Work out the finished part from the listing and answer in its coordinate system (mm). A direction names the side the tool comes from. Give positions to 0.01 mm unless a question says otherwise; leave off trailing zeros. Write each loop counter-clockwise with the first axis right and the second up, starting at its lowest first coordinate (ties: lowest second). Pieces come first, ordered by that corner, then holes. Notation, with made-up numbers: (19, -17) -> (39, -17) arc R27 cw to (39, 8) -> close; hole circle Ø2 at (59, 82). An arc over 180 degrees is marked (long way). Use a Markdown table: item, result. Add a question column.
Q1. For faces 1 (the face through (10.1, 1, 5)), 2 (the face through (12, -1, 10)), 3 (the face through (13.1, -1, 5)), 4 (the face through (-26.58, 5.75, 12.07)), 5 (the face through (-37, 38, 5)), determine the directions among +Z, -Z, +X, -X, +Y, -Y from which every point of the face is accessible in a straight line to the end or side of a thin tool.
Q2. Each of these flat-tipped pins is pushed along its axis until it touches: pin 1 Ø7 at (y, z) = (4, 14) entering from +X; pin 2 Ø4 at (y, z) = (5.1, 15) entering from -X; pin 3 Ø2 at (y, z) = (1, 4.5) entering from -X; pin 4 Ø12 at (y, z) = (40.5, 14.5) entering from -X. Where does it stop, or does it pass through?
Q3. For a pull along Z with two mould halves and no side action, classify faces 6 (the face through (-31.88, 4.56, 18.26)), 7 (the face through (-9.37, 5.17, 16.6)), 8 (the face through (-19, 3.8, 13.7)), 9 (the face through (5, 0, 8)) as pulls with the +Z half, pulls with the -Z half, needs draft (parallel to the pull), parting line crosses it, or undercut.
Q4. Section B-B, the plane x = -27 is taken. Give the vertices of the cut face in (y, z), plus the area to 3 significant figures.
Q5. Consider line 1 (Z direction, x = -23.5, y = 5.1); line 2 (Z direction, x = -6, y = 5); line 3 (Y direction, x = -9.75, z = 15). Determine where each line is inside the solid, lowest interval first.
Q6. Section A-A, the plane z = 6.25 is taken. Give the vertices of the cut face in (x, y), plus the area to 3 significant figures.
Q7. Section D-D, the plane z = 15 is taken. Give the vertices of the cut face in (x, y).
from build123d import *

# Parameters (mm, degrees)
EXTRUDE_1_DEPTH     = 10
SKETCH_2_W          = 30.142135624
SKETCH_2_H          = 14
EXTRUDE_2_DEPTH     = 10
CHAMFER_2_SIZE      = 10
SKETCH_3_R          = 1.6
CUT_EXTRUDE_1_DEPTH = 77.000065789
SKETCH_4_R          = 3
CUT_EXTRUDE_2_DEPTH = 23


with BuildPart() as part:
    # ｽｹｯﾁ1 → ﾎﾞｽ - 押し出し1 (new body)
    with BuildSketch(Plane.XY):
        Polygon((0, 0), (0, 10.1), (-30, 10.1), (-37, 17.1), (-37, 60.1), (-42, 60.1), (-42, 7.957864376), (-30.142135624, -3.9), (13.1, -3.9), (13.1, 2), (10.1, 2), (10.1, 0), align=None)
    extrude(amount=EXTRUDE_1_DEPTH)

    # ｽｹｯﾁ2 → ﾎﾞｽ - 押し出し2 (add)
    with BuildSketch(Plane.XY.offset(10)):
        with Locations((-15.071067812, 3.1)):
            Rectangle(SKETCH_2_W, SKETCH_2_H)
    extrude(amount=EXTRUDE_2_DEPTH)

    # 面取り2
    chamfer_2_edges = [part.edges().sort_by_distance(p)[0] for p in [
        (-30.142135624, 3.1, 10),
        (0, -1.95, 10),
    ]]
    chamfer(chamfer_2_edges, length=CHAMFER_2_SIZE - 0.0001)  # a hair under: the kernel refuses the full size

    # ｽｹｯﾁ3 → ｶｯﾄ - 押し出し1 (cut, through all)
    with BuildSketch(Plane(origin=(0, 0, 0), x_dir=(0, 0, -1), z_dir=(1, 0, 0))):
        with Locations((-15, 5.1)):
            Circle(SKETCH_3_R)
    extrude(amount=-CUT_EXTRUDE_1_DEPTH, mode=Mode.SUBTRACT)

    # ｽｹｯﾁ4 → ｶｯﾄ - 押し出し2 (cut)
    with BuildSketch(Plane.ZY.offset(42)):
        with Locations(Location((15, 5.1, 0), (0, 0, 270))):
            Circle(SKETCH_4_R)
    extrude(amount=-CUT_EXTRUDE_2_DEPTH, mode=Mode.SUBTRACT)


solid = part.part
Result set:
| question | item | result |
|---|---|---|
| 1 | face 1 | +Z, -Z, +Y |
| 1 | face 2 | +Z, +X, +Y, -Y |
| 1 | face 3 | +Z, -Z, +X, +Y, -Y |
| 1 | face 4 | -X |
| 1 | face 5 | +Z, -Z, +X, +Y |
| 2 | pin 1 | stops at x = 0 |
| 2 | pin 2 | stops at x = -19 |
| 2 | pin 3 | stops at x = -36.04 |
| 2 | pin 4 | stops at x = -42 |
| 3 | face 6 | pulls with the +Z half |
| 3 | face 7 | undercut |
| 3 | face 8 | undercut |
| 3 | face 9 | needs draft |
| 4 | outline | (-3.9, 0) -> (10.1, 0) -> (10.1, 20) -> (-3.9, 20) -> close; hole circle Ø6 at (5.1, 15) |
| 4 | area | 252 mm2 |
| 5 | line 1 | z = 0 to 12, 18 to 20 |
| 5 | line 2 | z = 0 to 13.4, 16.6 to 20 |
| 5 | line 3 | y = -3.9 to 3.5, 6.7 to 10.1 |
| 6 | outline | (-42, 7.96) -> (-30.14, -3.9) -> (13.1, -3.9) -> (13.1, 2) -> (10.1, 2) -> (10.1, 0) -> (0, 0) -> (0, 10.1) -> (-30, 10.1) -> (-37, 17.1) -> (-37, 60.1) -> (-42, 60.1) -> close |
| 6 | area | 849 mm2 |
| 7 | outline | (-35.14, 1.1) -> (-30.14, -3.9) -> (5, -3.9) -> (5, 0) -> (0, 0) -> (0, 3.5) -> (-19, 3.5) -> (-19, 2.1) -> (-35.14, 2.1) -> close; (-35.14, 8.1) -> (-19, 8.1) -> (-19, 6.7) -> (0, 6.7) -> (0, 10.1) -> (-35.14, 10.1) -> close |
